CAD build for the part. Positions are in the model's coordinates, mm. Round coordinates to 2 decimals unless told otherwise and drop trailing zeros. Write each loop counter-clockwise with the first axis right and the second up, starting at its lowest first coordinate (ties: lowest second). Pieces come first, ordered by that corner, then holes. Notation, with made-up numbers: (52, 30) -> (67, 30) arc R32 cw to (67, 65) -> close; hole circle Ø5 at (-7.75, -39). An arc over 180 degrees is marked (long way). Put each result on its own line as item: value. Start each with the question number.
1. Flat gauge pins, fed straight in: P1, Ø1.8, axis at x = -57.5, z = 21.5, coming from the -Y side; P2, Ø6, axis at y = 162.5, z = -8.5, coming from the +X side; P3, Ø1, axis at x = 41, y = 172, coming from the +Z side; P4, Ø8, axis at x = 0, y = 79.7, coming from the -Z side. Where does each tip first touch, or does it go through?
2. Saw through at B-B on z = -4.5. List the corners of the cut face in (x, y).
3. Saw through at A-A on y = 18. State how many separate pieces and enclosed holes the cut face has, and give its area (3 significant figures).
4. Pull direction X, two halves, no side cores. Call faces 1 (the cylindrical face through (-4.496, 79.898, 61.022)), 2 (the flat face through (-51, 101.6, 33)): pulls with the +X half, pulls with the -X half, needs draft (parallel to the pull), parting line crosses it, or undercut.
5. Drill centre lines: line 1 (Y direction, x = 0, z = 60.8); line 2 (X direction, y = 165.5, z = 0) (1 decimal); line 3 (X direction, y = 133, z = 14). Where is each one in solid material? Low to high. Write a range as from..to.
6. Saw through at C-C on x = -19.5. List the corners of the cut face in (y, z).
from build123d import *

# Parameters (mm, degrees)
CUT_EXTRUDE1_DEPTH      = 256.209705365
CUT_EXTRUDE1_DEPTH_BACK = 256.209705365
SKETCH2_R               = 4.5
CUT_EXTRUDE2_DEPTH      = 256.209705507
CIRPATTERN1_COUNT       = 4


with BuildPart() as part:
    # Sketch1 → Revolve1 (revolve)
    with BuildSketch(Plane.XY, mode=Mode.PRIVATE) as revolve1_sk:
        Polygon((-60.325, 239.72), (-60.325, 238.1325), (-60.325, 0), (-61.9125, 0), (-61.9125, 239.72), align=None)
    revolve(revolve1_sk.sketch.rotate(Axis((0, 0, 0), (0, 1, 0)), 270), axis=Axis((0, 0, 0), (0, 1, 0)))

    # Sketch2 → Cut-Extrude1 (cut, two sides: drawn at the far end of the back side and taken through both)
    with BuildSketch(Plane.XY.offset(-CUT_EXTRUDE1_DEPTH_BACK)):
        with Locations((0, 79.7)):
            Circle(SKETCH2_R)
    extrude(amount=CUT_EXTRUDE1_DEPTH + CUT_EXTRUDE1_DEPTH_BACK, mode=Mode.SUBTRACT)

    # Sketch3 → Cut-Extrude2 (cut, through all)
    with BuildSketch(Plane(origin=(0, 0, 0), x_dir=(0.906307787036651, 0, -0.4226182617406972), z_dir=(0.4226182617406972, 0, 0.906307787036651))):
        Polygon((-15.875, 0), (-15.875, 101.6), (-0.79375, 101.6), (-0.79375, 225.4325), (-25.4, 225.4325), (-25.4, 227.02), (25.4, 227.02), (25.4, 225.4325), (0.79375, 225.4325), (0.79375, 101.6), (15.875, 101.6), (15.875, 0), align=None)
    cut_extrude2 = extrude(amount=-CUT_EXTRUDE2_DEPTH, mode=Mode.SUBTRACT)

    # CirPattern1: Cut-Extrude2 ×4 about axis
    cirpattern1_axis = Axis((0, 0, 0), (0, 1, 0))
    for i in range(1, CIRPATTERN1_COUNT):
        add(cut_extrude2.rotate(cirpattern1_axis, i * 360 / CIRPATTERN1_COUNT), mode=Mode.SUBTRACT)


solid = part.part
Return value:
1. P1: stops at y = 101.6
1. P2: stops at x = 61.67
1. P3: stops at z = 46.83
1. P4: passes through
2. outline: (-61.75, 0) -> (-60.16, 0) -> (-60.16, 239.72) -> (-61.75, 239.72) -> close; (60.16, 0) -> (61.75, 0) -> (61.75, 225.43) -> (60.16, 225.43) -> close; (60.16, 227.02) -> (61.75, 227.02) -> (61.75, 239.72) -> (60.16, 239.72) -> close
3. separate pieces: 4
3. enclosed holes: 0
3. area: 406 mm^2
4. face 1: undercut
4. face 2: needs draft
5. line 1: y = 0..75.2, 84.2..239.72
5. line 2: x = -61.9..-60.3, 60.3..61.9
5. line 3: x = -60.31..-58.68, 58.68..60.31
6. outline: (0, 57.09) -> (239.72, 57.09) -> (239.72, 58.76) -> (0, 58.76) -> close; (101.6, -58.76) -> (225.43, -58.76) -> (225.43, -57.09) -> (101.6, -57.09) -> close; (227.02, -58.76) -> (239.72, -58.76) -> (239.72, -57.09) -> (227.02, -57.09) -> close
